Design review of the part built by this model. Coordinates are the model's own, in mm. A direction names the side the tool comes from. Round coordinates to 2 decimals unless told otherwise and drop trailing zeros. Order: outer loops, then holes, each group sorted by start corner. A loop starts at its lowest first (then second) coordinate and runs counter-clockwise, first axis right, second up. Notation, with made-up numbers: (5.5, 18.25) - (52.5, 18.25) arc R16 cw to (52.5, 27.25) - close; hole circle Ø6 at (75.25, 67). An arc over 180 degrees is marked (long way). Use CSV: the item, a comma, the result in double quotes.
from build123d import *

# Parameters (mm, degrees)
CYLINDER002_R     = 1
CYLINDER002_DEPTH = 10
ARRAY005_X_COUNT  = 2
ARRAY005_X_PITCH  = 66
ARRAY005_Y_COUNT  = 2
ARRAY005_Y_PITCH  = 46
BOX005_W          = 71
BOX005_H          = 51
BOX005_DEPTH      = 10
BOX004_W          = 67
BOX004_H          = 47
BOX004_DEPTH      = 10
BOX007_W          = 74
BOX007_H          = 54
BOX007_DEPTH      = 7.7
FILLET003_R       = 1.5
BOX006_W          = 7
BOX006_H          = 7
BOX006_DEPTH      = 6
FILLET002_R       = 1.5
ARRAY007_X_COUNT  = 2
ARRAY007_X_PITCH  = 64
ARRAY007_Y_COUNT  = 2
ARRAY007_Y_PITCH  = 44


with BuildPart() as dd_hole_array:
    # Cylinder002 → Cylinder002 (new body)
    with BuildSketch(Plane(origin=(4, 4, 0), x_dir=(1, 0, 0), z_dir=(0, 0, 1))):
        Circle(CYLINDER002_R)
    extrude(amount=CYLINDER002_DEPTH)

    # Array005 X: dd hole array ×2


with BuildPart() as dd_hole_array_1:
    add(dd_hole_array.part)
    with Locations(*[(i * ARRAY005_X_PITCH, 0, 0) for i in range(1, ARRAY005_X_COUNT)]):
        add(dd_hole_array.part)

    # Array005 Y: dd hole array ×2


with BuildPart() as dd_hole_array_2:
    add(dd_hole_array_1.part)
    with Locations(*[(0, i * ARRAY005_Y_PITCH, 0) for i in range(1, ARRAY005_Y_COUNT)]):
        add(dd_hole_array_1.part)


with BuildPart() as pcb_extraction001:
    # Box005 → Box005 (new body)
    with BuildSketch(Plane(origin=(1.5, 1.5, 5), x_dir=(1, 0, 0), z_dir=(0, 0, 1))):
        with Locations((35.5, 25.5)):
            Rectangle(BOX005_W, BOX005_H)
    extrude(amount=BOX005_DEPTH)


with BuildPart() as bottom_extraction003:
    # Box004 → Box004 (new body)
    with BuildSketch(Plane(origin=(3.5, 3.5, 0), x_dir=(1, 0, 0), z_dir=(0, 0, 1))):
        with Locations((33.5, 23.5)):
            Rectangle(BOX004_W, BOX004_H)
    extrude(amount=BOX004_DEPTH)

    # Fusion005: union pcb extraction001
    add(pcb_extraction001.part)


with BuildPart() as pcb_box_cut001:
    # Box007 → Box007 (new body)
    with BuildSketch(Plane.XY):
        with Locations((37, 27)):
            Rectangle(BOX007_W, BOX007_H)
    extrude(amount=BOX007_DEPTH)

    # Fillet003
    fillet003_edges = [pcb_box_cut001.edges().sort_by_distance(p)[0] for p in [
        (0, 0, 3.85),
        (0, 54, 3.85),
        (74, 0, 3.85),
        (74, 54, 3.85),
    ]]
    fillet(fillet003_edges, radius=FILLET003_R)

    # Cut002004: cut bottom extraction003
    add(bottom_extraction003.part, mode=Mode.SUBTRACT)


with BuildPart() as dd_frame_fusion_with_holes_no_attachment:
    # Box006 → Box006 (new body)
    with BuildSketch(Plane(origin=(1.5, 1.5, 0), x_dir=(1, 0, 0), z_dir=(0, 0, 1))):
        with Locations((3.5, 3.5)):
            Rectangle(BOX006_W, BOX006_H)
    extrude(amount=BOX006_DEPTH)

    # Fillet002
    fillet002_edges = [dd_frame_fusion_with_holes_no_attachment.edges().sort_by_distance(p)[0] for p in [
        (1.5, 1.5, 3),
        (1.5, 8.5, 3),
        (8.5, 1.5, 3),
        (8.5, 8.5, 3),
    ]]
    fillet(fillet002_edges, radius=FILLET002_R)

    # Array007 X: dd frame fusion with holes no attachment ×2


with BuildPart() as dd_frame_fusion_with_holes_no_attachment_1:
    add(dd_frame_fusion_with_holes_no_attachment.part)
    with Locations(*[(i * ARRAY007_X_PITCH, 0, 0) for i in range(1, ARRAY007_X_COUNT)]):
        add(dd_frame_fusion_with_holes_no_attachment.part)

    # Array007 Y: dd frame fusion with holes no attachment ×2


with BuildPart() as dd_frame_fusion_with_holes_no_attachment_2:
    add(dd_frame_fusion_with_holes_no_attachment_1.part)
    with Locations(*[(0, i * ARRAY007_Y_PITCH, 0) for i in range(1, ARRAY007_Y_COUNT)]):
        add(dd_frame_fusion_with_holes_no_attachment_1.part)

    # Fusion003: union pcb box cut001
    add(pcb_box_cut001.part)

    # Cut002005: cut dd hole array
    add(dd_hole_array_2.part, mode=Mode.SUBTRACT)


solid = dd_frame_fusion_with_holes_no_attachment_2.part
1) To check wall thickness, follow L1, parallel to Y at x = 70, z = 3.1; L2, parallel to X at y = 50, z = 3.55; L3, parallel to X at y = 42.5, z = 2.5. State the ranges of each line that lie inside material, in increasing order. Write a range as from..to.
Data:
L1,"y = 0..3, 5..8.5, 45.5..49, 51..54"
L2,"x = 0..3, 5..8.5, 65.5..69, 71..74"
L3,"x = 0..3.5, 70.5..74"
2) We need section B-B (z = 2.5). Give the boundary of the cut face in (x, y), then the cut area to 3 significant figures.
Data:
outline,"(0, 1.5) arc R1.5 ccw to (1.5, 0) - (72.5, 0) arc R1.5 ccw to (74, 1.5) - (74, 52.5) arc R1.5 ccw to (72.5, 54) - (1.5, 54) arc R1.5 ccw to (0, 52.5) - close; hole circle Ø2 at (4, 4); hole circle Ø2 at (4, 50); hole (3.5, 8.5) - (7, 8.5) arc R1.5 cw to (8.5, 7) - (8.5, 3.5) - (65.5, 3.5) - (65.5, 7) arc R1.5 cw to (67, 8.5) - (70.5, 8.5) - (70.5, 45.5) - (67, 45.5) arc R1.5 cw to (65.5, 47) - (65.5, 50.5) - (8.5, 50.5) - (8.5, 47) arc R1.5 cw to (7, 45.5) - (3.5, 45.5) - close; hole circle Ø2 at (70, 4); hole circle Ø2 at (70, 50)"
area,"931 mm2"
3) We need section C-C (x = 25). Give the boundary of the cut face in (y, z).
Data:
outline,"(0, 0) - (3.5, 0) - (3.5, 5) - (1.5, 5) - (1.5, 7.7) - (0, 7.7) - close; (50.5, 0) - (54, 0) - (54, 7.7) - (52.5, 7.7) - (52.5, 5) - (50.5, 5) - close"
4) For faces 1 (the face through (0.43, 53.55, 3.9)), 2 (the face through (37, 52, 5)), 3 (the face through (3.5, 27, 2)), list the 3-axis set-ups (+Z, -Z, +X, -X, +Y, -Y) from which the entire face can be reached by the end or side of a thin tool; tool diameter is ignored.
Data:
face 1,"+Z, -Z, -X, +Y"
face 2,"+Z"
face 3,"+Z, -Z"
5) Insertion check: pin 1 Ø1.2 at (x, y) = (2.5, 2.5) entering from +Z; pin 2 Ø1.8 at (x, y) = (70, 50) entering from +Z. Each pin has a flat end and moves straight along its axis. Give the tip position at first contact, or say it passes through.
Data:
pin 1,"stops at z = 6"
pin 2,"passes through"
6) We need section A-A (y = 30). Give the boundary of the cut face in (x, z), then the cut area to 3 significant figures.
Data:
outline,"(0, 0) - (3.5, 0) - (3.5, 5) - (1.5, 5) - (1.5, 7.7) - (0, 7.7) - close; (70.5, 0) - (74, 0) - (74, 7.7) - (72.5, 7.7) - (72.5, 5) - (70.5, 5) - close"
area,"43.1 mm2"
